Autodesk Inventor part; units mm, degrees
ref_plane "YZ Plane" through (0, 0, 0) normal (1, 0, 0) x (0, 1, 0)
ref_plane "XZ Plane" through (0, 0, 0) normal (0, 1, 0) x (-1, 0, 0)
ref_plane "XY Plane" through (0, 0, 0) normal (0, 0, 1) x (1, 0, 0)
ref_plane "Work Plane1" through (0, 0, 0) normal (0, 0, 1) x (1, 0, 0)
sketch "Sketch1" plane through (0, 0, 0) normal (0, 0, 1) x (1, 0, 0)
  circle A0 centre (0, 80) radius 1.8
  circle A1 centre (0, 11.4286) radius 1.8
  circle A2 centre (0, -34.2857) radius 1.8
  circle A3 centre (0, -80) radius 1.8
  circle A4 centre (0, -57.1429) radius 1.8
  circle A5 centre (0, -11.4286) radius 1.8
  circle A6 centre (0, 57.1429) radius 1.8
  circle A7 centre (0, 34.2857) radius 1.8
  line L0 (-3, 83) -> (3, 83)
  line L1 (-3, -83) -> (-3, 83)
  line L2 (3, -83) -> (-3, -83)
  line L3 (3, -83) -> (3, 83)
  point P0 (0, 0)
extrude "Extrusion1" add sketch "Sketch1" along normal blind 3
sketch "Sketch2" plane through (0, 0, 3) normal (0, 0, 1) x (1, 0, 0)
  point P0 (0, 0)
fillet "Fillet1" radius 1 4 edges at (3, 83, 1.5) (-3, 83, 1.5) (-3, -83, 1.5) (3, -83, 1.5)
properties part number "petg_holder_2"
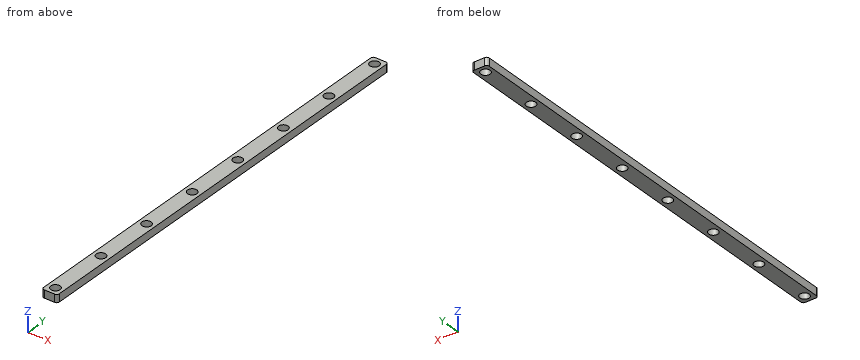
Part model, mm, in its own coordinate system. Round coordinates to 2 decimals unless told otherwise and drop trailing zeros. Loops run counter-clockwise (first coordinate to the right, second up) from the corner with the lowest first, then second, coordinate; pieces in that order, holes last. Notation, with made-up numbers: (-20.75, 72) -> (-4.75, 72) arc R24 ccw to (-4.75, 90) -> close; hole circle Ø4 at (88.5, -28). An arc over 180 degrees is marked (long way). Use one line per item in the form item = value. Start each with the question number.
Item 1: Band-saw the part on A-A (y = -80). List the corners of the cut face in (x, z).
Item 2: Band-saw the part on B-B (z = 0.75). Give the number of separate pieces and of enclosed holes in the cut face, plus the area to 3 significant figures.
Item 3: Drop a flat-ended pin along its axis: pin 1 Ø2 at (x, y) = (-2, -61.5) entering from -Z. Give the stop position or say it passes through.
Item 4: Drill centre lines: line 1 along Y through (x, z) = (-2.1, 1.8); line 2 along X through (y, z) = (-58, 2.6); line 3 along Y through (x, z) = (-2.5, 1). Where is each one in solid material? Low to high.
Data:
q1.outline = (-3, 0) -> (-1.8, 0) -> (-1.8, 3) -> (-3, 3) -> close; (1.8, 0) -> (3, 0) -> (3, 3) -> (1.8, 3) -> close
q2.separate_pieces = 1
q2.enclosed_holes = 8
q2.area = 914 mm^2
q3.pin_1 = 0
q4.line_1 = -82.99 to 82.99
q4.line_2 = -3 to -1.58, 1.58 to 3
q4.line_3 = -82.87 to 82.87
